Part model, mm, in its own coordinate system. A direction names the side the tool comes from. Round coordinates to 2 decimals unless told otherwise and drop trailing zeros. Loops run counter-clockwise (first coordinate to the right, second up) from the corner with the lowest first, then second, coordinate; pieces in that order, holes last. Notation, with made-up numbers: M 20,76.5 L 50,76.5 A21 ccw 50,106.5 Z; hole C 39,-24.75 d2. An arc over 180 degrees is marked long. Put each result on its own line as item: value. Start each with the question number.
1) Slice it at B-B on x = 19.5. Give the cut face in (y, z).
2) Pull direction X, two halves, no side cores. Call faces 3 (the flat face through (13, 6, -73.66)), 4 (the cylindrical face through (12.369, 6.439, -66.653)), 5 (the flat face through (25.4, 58, -21)): +X half, -X half, draft (parallel to the pull), parting line (faces both ways), or undercut.
3) Drop flat-ended pins along their axis: pin 1 Ø5.5 at (x, z) = (7.5, -60.5) entering from +Y; pin 2 Ø1 at (x, y) = (22, 116.5) entering from -Z; pin 3 Ø3 at (x, y) = (12.7, 136.525) entering from +Z; pin 4 Ø9.5 at (x, y) = (12, 133) entering from -Z. Give the stop position or say it passes through.
4) Slice it at A-A on x = 12.7. Give the cut face in (y, z) (3 decimals).
5) Slice it at C-C on z = -38. Give the cut face in (x, y), then the cut area to 3 significant figures.
6) Which spindle directions (+Z, -Z, +X, -X, +Y, -Y) get a long thin tool onto all of the face, cutting with end or side? Do faces 1 (the cylindrical face through (13.031, 139.043, -6.439)), 2 (the flat face through (10, 12.7, -64)). Say none if no direction does.
7) Probe line 1 along Y through (x, z) = (12.7, -7.25) (3 decimals); line 2 along Z through (x, y) = (12.7, 7.5) (3 decimals); line 3 along Y through (x, z) = (11.25, -66.5). List the from-to ranges inside material, lowest first.
8) Slice it at D-D on y = 25. Give the cut face in (x, z), then the cut area to 3 significant figures.
```python
from build123d import *

# Parameters (mm, degrees)
BOSS_EXTRUDE1_DEPTH = 25.4
SKETCH2_R           = 2.54
CUT_EXTRUDE1_DEPTH  = 13.7
SKETCH3_R           = 2.54
CUT_EXTRUDE2_DEPTH  = 13.7


with BuildPart() as part:
    # Sketch1 → Boss-Extrude1 (new body)
    with BuildSketch(Plane(origin=(0, 0, 0), x_dir=(0, 0, -1), z_dir=(1, 0, 0))):
        Polygon((0, 0), (0, 146.05), (12.7, 146.05), (12.7, 127), (54.61, 12.7), (73.66, 12.7), (73.66, 0), align=None)
    extrude(amount=BOSS_EXTRUDE1_DEPTH)

    # Sketch2 → Cut-Extrude1 (cut, through all)
    with BuildSketch(Plane(origin=(0, 0, -12.7), x_dir=(-1, 0, 0), z_dir=(0, 0, -1))):
        with Locations((-12.7, 136.525)):
            Circle(SKETCH2_R)
    extrude(amount=-CUT_EXTRUDE1_DEPTH, mode=Mode.SUBTRACT)

    # Sketch3 → Cut-Extrude2 (cut, through all)
    with BuildSketch(Plane(origin=(0, 12.7, 0), x_dir=(1, 0, 0), z_dir=(0, 1, 0))):
        with Locations((12.7, 64.135)):
            Circle(SKETCH3_R)
    extrude(amount=-CUT_EXTRUDE2_DEPTH, mode=Mode.SUBTRACT)


solid = part.part
```
Recorded:
1. outline: M 0,-73.66 L 12.7,-73.66 L 12.7,-54.61 L 127,-12.7 L 146.05,-12.7 L 146.05,0 L 0,0 Z
2. face 3: draft
2. face 4: undercut
2. face 5: +X half
3. pin 1: stops at y = 12.7
3. pin 2: stops at z = -16.73
3. pin 3: passes through
3. pin 4: stops at z = -12.7
4. outline: M 0,-73.66 L 12.7,-73.66 L 12.7,-66.675 L 0,-66.675 Z; M 0,-61.595 L 12.7,-61.595 L 12.7,-54.61 L 127,-12.7 L 133.985,-12.7 L 133.985,0 L 0,0 Z; M 139.065,-12.7 L 146.05,-12.7 L 146.05,0 L 139.065,0 Z
5. outline: M 0,0 L 25.4,0 L 25.4,58 L 0,58 Z
5. area: 1,470 mm2
6. face 1: +Z, -Z
6. face 2: -Z, +X, -X, +Y
7. line 1: y = 0 to 133.985, 139.065 to 146.05
7. line 2: z = -73.66 to -66.675, -61.595 to 0
7. line 3: y = 0 to 12.7
8. outline: M 0,-50.1 L 25.4,-50.1 L 25.4,0 L 0,0 Z
8. area: 1,270 mm2
